Input: dimensioned drawing with shaded views. Units: mm. Origin: part minimum x, y, z. A direction names the side the tool comes from. Coordinates: 2 decimals unless noted, no trailing zeros. Order: outer loops, then holes, each group sorted by start corner. A loop starts at its lowest first (then second) coordinate and runs counter-clockwise, first axis right, second up.
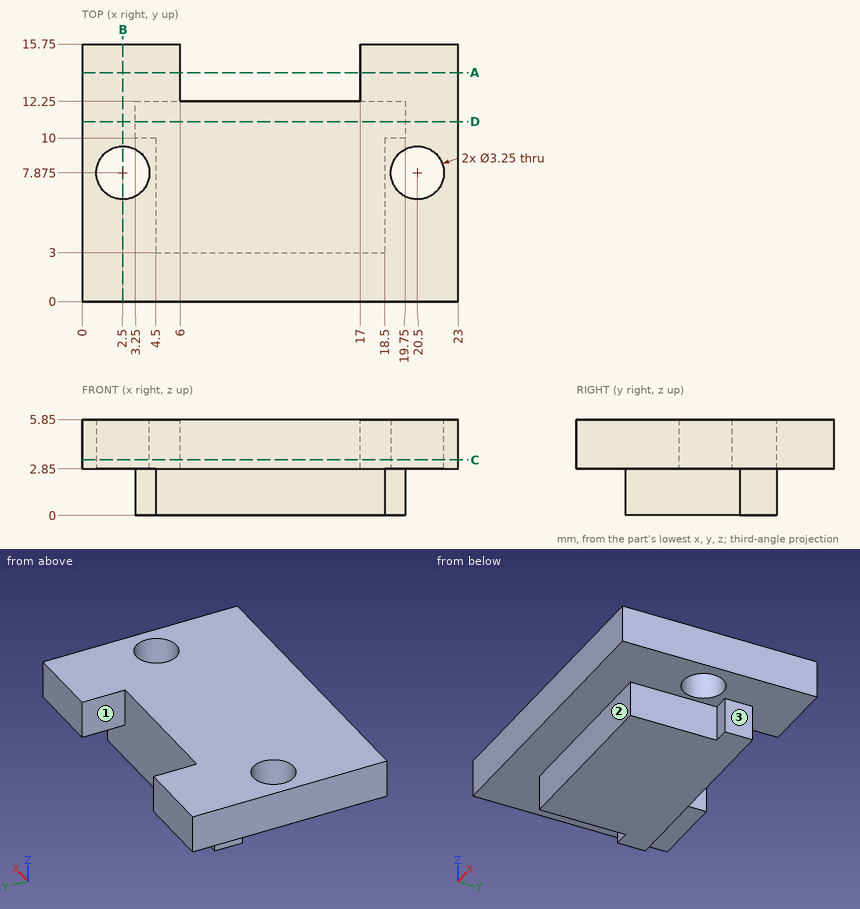
1. Access query for the marked faces 1, 2 and 3. Directions: +Z, -Z, +X, -X, +Y, -Y. A direction counts if a zero-diameter tool reaches every point of the face in a straight line with its end or side. Return the directions, or none.
2. Section query A-A, the plane y = 14. Output: boundary loops of the cut face in (x, z).
3. Section query B-B, the plane x = 2.5. Output: boundary loops of the cut face in (y, z).
4. Section query C-C, the plane z = 3.4. Output: boundary loops of the cut face in (x, y) (3 decimals), plus the area to 3 significant figures.
5. Section query D-D, the plane y = 11. Output: boundary loops of the cut face in (x, z), plus the area to 3 significant figures.
6. Contact query for flat-ended pins moving along their axis: P1, Ø2.5, axis at y = 10.5, z = 1.5, coming from the +X side; P2, Ø1.4, axis at x = 4, z = 1, coming from the -Y side; P3, Ø1.1, axis at y = 11.5, z = 1, coming from the -X side. Output: stop coordinate, or through.
7. Material intervals for line 1 along X through (y, z) = (15.25, 4.8); line 2 along Y through (x, z) = (2.5, 4.65); line 3 along X through (y, z) = (8.25, 4.05), sorted ascending.
Answer key:
1. face 1: +Z, -Z, +Y
1. face 2: -Z, +X, -X, -Y
1. face 3: -Z, +X, +Y, -Y
2. outline: (0, 2.85) - (6, 2.85) - (6, 5.85) - (0, 5.85) - close; (17, 2.85) - (23, 2.85) - (23, 5.85) - (17, 5.85) - close
3. outline: (0, 2.85) - (6.25, 2.85) - (6.25, 5.85) - (0, 5.85) - close; (9.5, 2.85) - (15.75, 2.85) - (15.75, 5.85) - (9.5, 5.85) - close
4. outline: (0, 0) - (23, 0) - (23, 15.75) - (17, 15.75) - (17, 12.25) - (6, 12.25) - (6, 15.75) - (0, 15.75) - close; hole circle Ø3.25 at (2.5, 7.875); hole circle Ø3.25 at (20.5, 7.875)
4. area: 307 mm2
5. outline: (0, 2.85) - (3.25, 2.85) - (3.25, 0) - (19.75, 0) - (19.75, 2.85) - (23, 2.85) - (23, 5.85) - (0, 5.85) - close
5. area: 116 mm2
6. P1: stops at x = 19.75
6. P2: stops at y = 3
6. P3: stops at x = 3.25
7. line 1: x = 0 to 6, 17 to 23
7. line 2: y = 0 to 6.25, 9.5 to 15.75
7. line 3: x = 0 to 0.92, 4.08 to 18.92, 22.08 to 23
